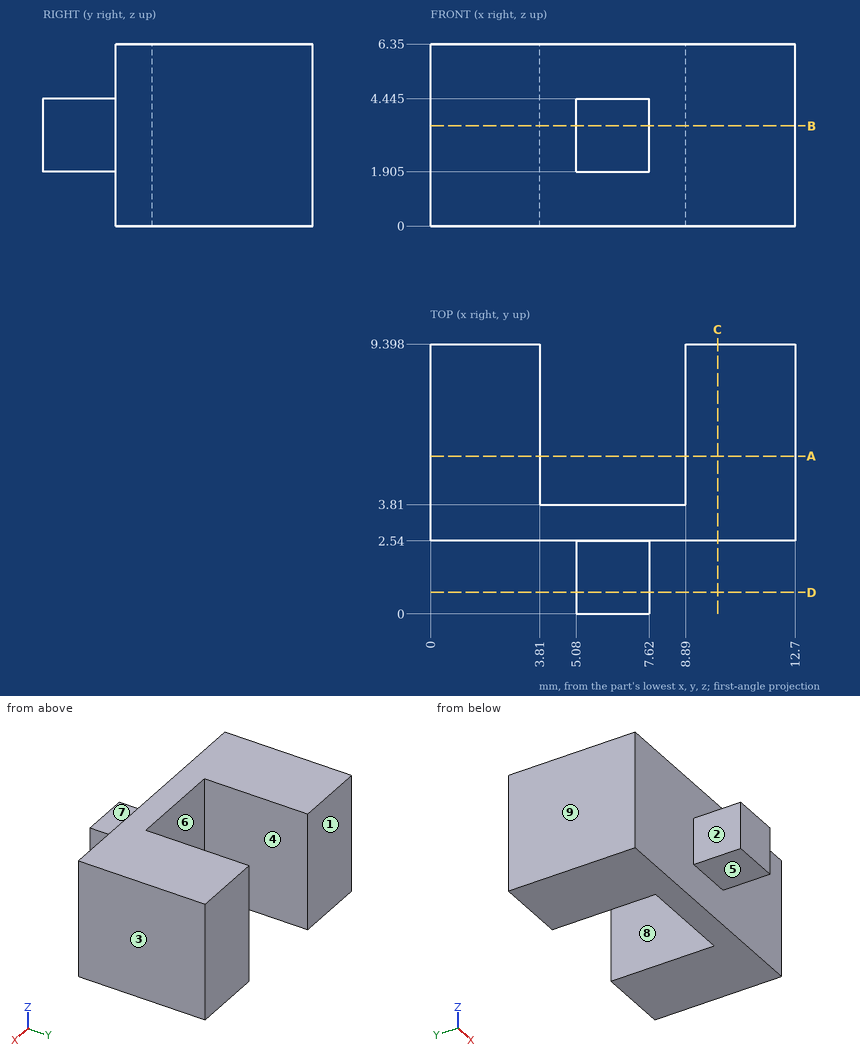
Job drawing, mm, ordinate dimensions from the low corner. One solid piece. A direction names the side the tool comes from. Give positions to 0.01 mm unless a question says otherwise; leave off trailing zeros. Loops run counter-clockwise (first coordinate to the right, second up) from the corner with the lowest first, then second, coordinate; pieces in that order, holes last. Notation, with made-up numbers: M -16,-33.5 L 24,-33.5 A21 cw 24,-2.5 Z; hole C 63,3 d6. An arc over 180 degrees is marked long. Return JSON: item names as keys, results as strings.
1) Drill centre lines: line 1 (X direction, y = 7.75, z = 5.25); line 2 (Y direction, x = 5, z = 5.75); line 3 (Y direction, x = 11.75, z = 2.5). Where is each one in solid material? Low to high.
Calculated:
{"line 1": "x = 0 to 3.81, 8.89 to 12.7", "line 2": "y = 2.54 to 3.81", "line 3": "y = 2.54 to 9.4"}
2) Saw through at A-A, the plane y = 5.5. List the corners of the cut face in (x, z), then the cut area to 3 significant figures.
Calculated:
{"outline": "M 0,0 L 3.81,0 L 3.81,6.35 L 0,6.35 Z; M 8.89,0 L 12.7,0 L 12.7,6.35 L 8.89,6.35 Z", "area": "48.4 mm2"}
3) Pull direction X, two halves, no side cores. Call the marked faces 6, 7, 8 and 9: released by +X, released by -X, zero draft, split by the parting line, or undercut.
Calculated:
{"face 6": "undercut", "face 7": "zero draft", "face 8": "undercut", "face 9": "released by -X"}
4) Saw through at B-B, the plane z = 3.5. List the corners of the cut face in (x, y).
Calculated:
{"outline": "M 0,2.54 L 5.08,2.54 L 5.08,0 L 7.62,0 L 7.62,2.54 L 12.7,2.54 L 12.7,9.4 L 8.89,9.4 L 8.89,3.81 L 3.81,3.81 L 3.81,9.4 L 0,9.4 Z"}
5) 3-axis set-ups, long thin cutter, end or side, ignore diameter. For the marked faces 1, 2, 3, 4 and 5: which of +Z, -Z, +X, -X, +Y, -Y reach the whole face in a straight line?
Calculated:
{"face 1": "+Z, -Z, +X, -X, +Y", "face 2": "+Z, -Z, -X, -Y", "face 3": "+Z, -Z, +X, +Y, -Y", "face 4": "+Z, -Z, +Y", "face 5": "-Z, +X, -X, -Y"}
6) Flat gauge pins, fed straight in: pin 1 Ø2 at (x, y) = (4.5, 3.5) entering from -Z; pin 2 Ø3 at (y, z) = (1, 2.5) entering from +X; pin 3 Ø0.8 at (x, y) = (6.5, 1.5) entering from +Z (3 decimals); pin 4 Ø2 at (x, y) = (6.5, 1.5) entering from -Z (3 decimals). Where does each tip first touch, or does it go through?
Calculated:
{"pin 1": "stops at z = 0", "pin 2": "stops at x = 7.62", "pin 3": "stops at z = 4.445", "pin 4": "stops at z = 1.905"}
7) Saw through at D-D, the plane y = 0.75. List the corners of the cut face in (x, z) (3 decimals).
Calculated:
{"outline": "M 5.08,1.905 L 7.62,1.905 L 7.62,4.445 L 5.08,4.445 Z"}
8) Saw through at C-C, the plane x = 10. List the corners of the cut face in (y, z).
Calculated:
{"outline": "M 2.54,0 L 9.4,0 L 9.4,6.35 L 2.54,6.35 Z"}
